Can you work these out from the model? Positions are in its coordinate system, mm. A direction names the side the tool comes from. Coordinates: 2 decimals unless noted, no trailing zeros. Write each loop counter-clockwise with the first axis right and the second up, starting at its lowest first coordinate (ties: lowest second). Pieces come first, ordered by that corner, then holes. Notation, with made-up numbers: M -35,11 L 4,11 A6 cw 4,19 Z; hole C -0.75,28 d2. An arc over 180 degrees is marked long. Use one line per item in the form item = value. Start each with the question number.
```python
from build123d import *

# Parameters (mm, degrees)
F0_R     = 11.25
F0_R_2   = 8.25
F1_DEPTH = 11
F2_R     = 8.25
F3_DEPTH = 9
F4_R     = 8.5
F4_R_2   = 7.5
F5_DEPTH = 13


with BuildPart() as f1:
    # F0 (on Front) → F1 (new body)
    with BuildSketch(Plane.XZ):
        Circle(F0_R)
        Circle(F0_R_2, mode=Mode.SUBTRACT)
    extrude(amount=F1_DEPTH)

    # F2 (on face) → F3 (join)
    with BuildSketch(Plane.XZ.offset(11)):
        Polygon((6.495191, 11.25), (-6.495191, 11.25), (-12.990381, 0), (-6.495191, -11.25), (6.495191, -11.25), (12.990381, 0), align=None)
        Circle(F2_R, mode=Mode.SUBTRACT)
    extrude(amount=F3_DEPTH)

    # F4 (on face) → F5 (join)
    with BuildSketch(Plane.XZ.offset(20)):
        Circle(F4_R)
        Circle(F4_R_2, mode=Mode.SUBTRACT)
    extrude(amount=F5_DEPTH)

    # F6 (on Top) → F7 (revolve)
    with BuildSketch(Plane.XY):
        with BuildLine():
            Line((7.544115, -39), (8.5, -39))
            ThreePointArc((8.5, -39), (11.5, -36), (8.5, -33))
            Line((8.5, -33), (7.544115, -33))
            Line((7.544115, -33), (7.544115, -39))
        make_face()
    revolve(axis=Axis((0, -35.327807, 0), (0, 1, 0)))


solid = f1.part
```
1) Please list where these lines run through material, in increasing order: line 1 (Z direction, x = 0, y = -28.5); line 2 (Y direction, x = 9.25, z = -4.25); line 3 (X direction, y = -22, z = -3).
2) Will these pins go through, and if not, where does the flat tip stop? pin 1 Ø7 at (x, y) = (-1, -13.5) entering from -Z; pin 2 Ø13.5 at (x, z) = (0, 0) entering from -Y; pin 3 Ø7 at (x, y) = (1.5, -16.5) entering from +Z; pin 4 Ø4 at (x, y) = (4, -32) entering from +Z.
3) If we mould it in two halves opening along X, with no side actions, what happens to faces 4 (the face through (9.788, -15.437, 5.546)), 5 (the face through (7.62, -9.86, -3.16)), 6 (the face through (-12, -11, 0))? For each: +X half, -X half, draft (parallel to the pull), parting line (faces both ways), or undercut.
4) Which directions (+Z, -Z, +X, -X, +Y, -Y) give clear straight access to the entire face, cutting with the end or side of a thin tool? Please do faces 1 (the face through (6, -11, -10)), 2 (the face through (-9.788, -15.437, -5.546)), 3 (the face through (4.57, -26.409, 7.167)).
5) Suppose I cut it at B-B on y = -31. Please give me the cut outline in (x, z), and give its area (3 significant figures).
6) Suppose I cut it at A-A on y = -16.5. Please give me the cut outline in (x, z), and give its area (3 significant figures).
Computed values:
q1.line_1 = -8.5 to -7.5, 7.5 to 8.5
q1.line_2 = -38.49 to -33.51, -20 to 0
q1.line_3 = -7.95 to -6.87, 6.87 to 7.95
q2.pin_1 = -11.25
q2.pin_2 = through
q2.pin_3 = 11.25
q2.pin_4 = 10.09
q3.face_4 = +X half
q3.face_5 = undercut
q3.face_6 = draft
q4.face_1 = -Z, +X, +Y
q4.face_2 = -Z, -X, +Y
q4.face_3 = none
q5.outline = C 0,0 d17; hole C 0,0 d15
q5.area = 50.3 mm²
q6.outline = M -12.99,0 L -6.5,-11.25 L 6.5,-11.25 L 12.99,0 L 6.5,11.25 L -6.5,11.25 Z; hole C 0,0 d16.5
q6.area = 225 mm²
